Could you check a few things on this drawing? It's one solid part, dimensions in mm from its lowest x, y, z. A direction names the side the tool comes from. Give positions to 0.01 mm unless a question says otherwise; leave off trailing zeros. Loops run counter-clockwise (first coordinate to the right, second up) from the corner with the lowest first, then second, coordinate; pieces in that order, holes last. Notation, with made-up numbers: (85, 47.25) - (141, 47.25) arc R31 ccw to (141, 81.25) - close; hole circle Ø1 at (1.25, 54.25). An arc over 180 degrees is marked (long way). Use a Markdown table: item, result.
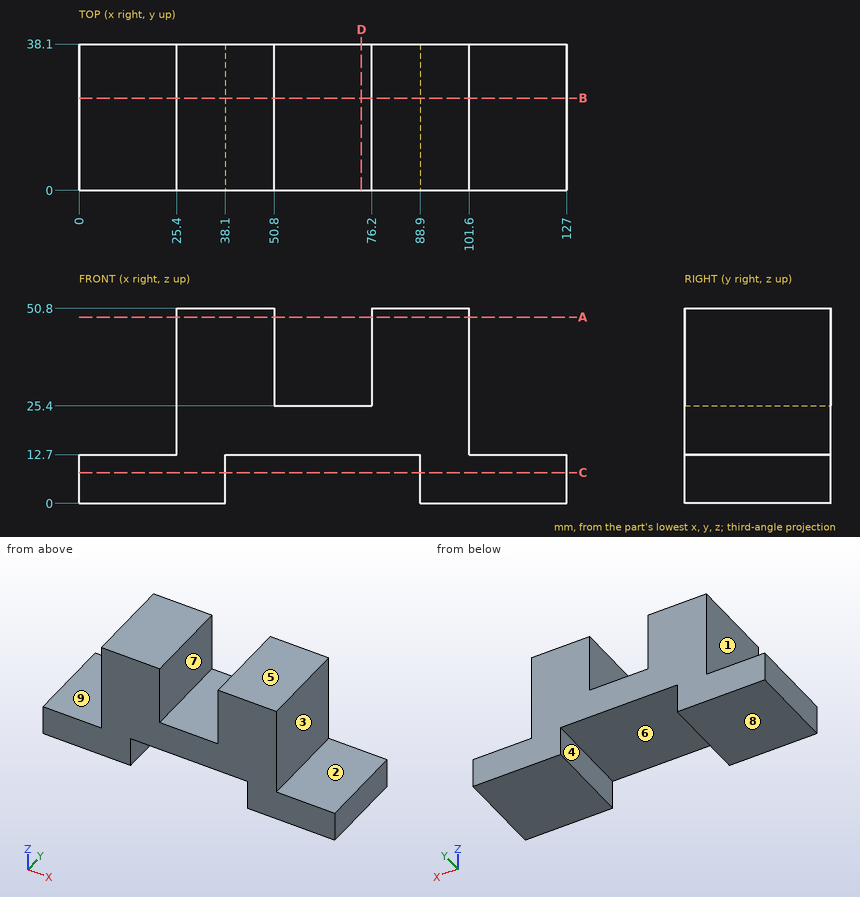
(1) If I drill on line 1 (X direction, y = 13.5, z = 3); line 2 (X direction, y = 8, z = 37); line 3 (Z direction, x = 17.5, y = 23.5), over which ranges is the centre line in solid material (lowest first)?
A:
| item | result |
|---|---|
| line 1 | 0 to 38.1, 88.9 to 127 |
| line 2 | 25.4 to 50.8, 76.2 to 101.6 |
| line 3 | 0 to 12.7 |
(2) Suppose I cut it at A-A on z = 48.5. Write out the boundary of the cut face in (x, y), plus the area to 3 significant figures.
A:
| item | result |
|---|---|
| outline | (25.4, 0) - (50.8, 0) - (50.8, 38.1) - (25.4, 38.1) - close; (76.2, 0) - (101.6, 0) - (101.6, 38.1) - (76.2, 38.1) - close |
| area | 1,940 mm2 |
(3) Suppose I cut it at B-B on y = 24. Write out the boundary of the cut face in (x, z), plus the area to 3 significant figures.
A:
| item | result |
|---|---|
| outline | (0, 0) - (38.1, 0) - (38.1, 12.7) - (88.9, 12.7) - (88.9, 0) - (127, 0) - (127, 12.7) - (101.6, 12.7) - (101.6, 50.8) - (76.2, 50.8) - (76.2, 25.4) - (50.8, 25.4) - (50.8, 50.8) - (25.4, 50.8) - (25.4, 12.7) - (0, 12.7) - close |
| area | 3,230 mm2 |
(4) We'd pull the mould along X, two halves only. Please class the marked faces 1, 2, 3 and 4: pulls with the +X half, pulls with the -X half, needs draft (parallel to the pull), parting line crosses it, or undercut.
A:
| item | result |
|---|---|
| face 1 | pulls with the -X half |
| face 2 | needs draft |
| face 3 | pulls with the +X half |
| face 4 | undercut |
(5) Suppose I cut it at D-D on x = 73.5. Write out the boundary of the cut face in (y, z).
A:
| item | result |
|---|---|
| outline | (0, 12.7) - (38.1, 12.7) - (38.1, 25.4) - (0, 25.4) - close |
(6) Will these pins go through, and if not, where does the flat tip stop? pin 1 (1.5 mm diameter, centred on y = 32, z = 43.5, fed in from +X); pin 2 (12.5 mm diameter, centred on x = 117.5, y = 24.5, fed in from +Z); pin 3 (12.5 mm diameter, centred on x = 69.5, y = 16, fed in from +Z).
A:
| item | result |
|---|---|
| pin 1 | x = 101.6 |
| pin 2 | z = 12.7 |
| pin 3 | z = 25.4 |
(7) Suppose I cut it at C-C on z = 8. Write out the boundary of the cut face in (x, y).
A:
| item | result |
|---|---|
| outline | (0, 0) - (38.1, 0) - (38.1, 38.1) - (0, 38.1) - close; (88.9, 0) - (127, 0) - (127, 38.1) - (88.9, 38.1) - close |
(8) On a 3-axis mill with a long thin cutter (end or side, diameter ignored), from which of +Z, -Z, +X, -X, +Y, -Y can I reach the whole of each face in a straight line? I mean the marked faces 5, 6, 7, 8 and 9. Say none if no direction works.
A:
| item | result |
|---|---|
| face 5 | +Z, +X, -X, +Y, -Y |
| face 6 | -Z, +Y, -Y |
| face 7 | +Z, +Y, -Y |
| face 8 | -Z, +X, -X, +Y, -Y |
| face 9 | +Z, -X, +Y, -Y |
